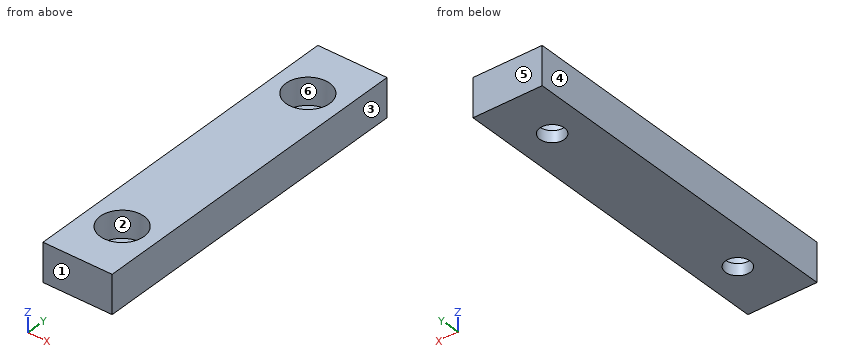
```python
from build123d import *

# Parameters (mm, degrees)
SKETCH1_W           = 44.4
SKETCH1_H           = 9
SKETCH1_R           = 2.85
BOSS_EXTRUDE1_DEPTH = 5
SKETCH1_3_R         = 2.85
SKETCH1_3_R_2       = 1.6
BOSS_EXTRUDE2_DEPTH = 1.5


with BuildPart() as part:
    # Sketch1 → Boss-Extrude1 (new body)
    with BuildSketch(Plane(origin=(0, 0, 0), x_dir=(0, 1, 0), z_dir=(0, 0, 1))):
        Rectangle(SKETCH1_W, SKETCH1_H)
        with Locations((15, 0)):
            Circle(SKETCH1_R, mode=Mode.SUBTRACT)
        with Locations((-15, 0)):
            Circle(SKETCH1_R, mode=Mode.SUBTRACT)
    extrude(amount=BOSS_EXTRUDE1_DEPTH)

    # Sketch1_3 → Boss-Extrude2 (add)
    with BuildSketch(Plane(origin=(0, 0, 0), x_dir=(0, 1, 0), z_dir=(0, 0, 1))):
        with Locations((15, 0)):
            Circle(SKETCH1_3_R)
        with Locations((15, 0)):
            Circle(SKETCH1_3_R_2, mode=Mode.SUBTRACT)
        with Locations((-15, 0)):
            Circle(SKETCH1_3_R)
        with Locations((-15, 0)):
            Circle(SKETCH1_3_R_2, mode=Mode.SUBTRACT)
    extrude(amount=BOSS_EXTRUDE2_DEPTH)


solid = part.part
```
Check sheet for the modelled part. Datum: model origin and axes. Units: mm. Face numbers are marked on the shaded views. A direction names the side the tool comes from. Give positions to 0.01 mm unless a question says otherwise; leave off trailing zeros. Write each loop counter-clockwise with the first axis right and the second up, starting at its lowest first coordinate (ties: lowest second). Pieces come first, ordered by that corner, then holes. Notation, with made-up numbers: (8, 55) - (54, 55) arc R27 ccw to (54, 88) - close; hole circle Ø3 at (31, 10.25). An arc over 180 degrees is marked (long way). Answer as a JSON object with one key per item and string values. Group by question number.
1) Depth check by flat-ended pin: P1, Ø3, axis at x = -1, y = -15, coming from the +Z side. Enter the tip coordinate at first touch or a pass-through.
2) Sectioned sample at C-C (z = 2.6). Record the cut outline in (x, y).
3) Thickness scan on probe 1 along Y at (x, z) = (0, 4.1); probe 2 along Y at (x, z) = (0, 0.8); probe 3 along X at (y, z) = (-15, 1.15). Record the ranges inside material, lowest first. Write a range as from..to.
4) Sectioned sample at B-B (y = 15). Record the cut outline in (x, z), then the cut area to 4 significant figures.
5) Access from +Z, -Z, +X, -X, +Y, -Y to the whole of each face (thin tool, end or side, straight path). Record for the marked faces 5 and 6.
6) Release check for a two-part mould opening along X. For the marked faces 1, 2, 3 and 4 record: pulls with the +X half, pulls with the -X half, needs draft (parallel to the pull), parting line crosses it, or undercut.
7) Sectioned sample at D-D (y = -14.5). Record the cut outline in (x, z), then the cut area to 3 significant figures.
8) Sectioned sample at A-A (x = 0). Record the cut outline in (y, z), then the cut area to 4 significant figures.
Geometry results:
{
 "1": {"P1": "stops at z = 1.5"},
 "2": {"outline": "(-4.5, -22.2) - (4.5, -22.2) - (4.5, 22.2) - (-4.5, 22.2) - close; hole circle Ø5.7 at (0, -15); hole circle Ø5.7 at (0, 15)"},
 "3": {"probe 1": "y = -22.2..-17.85, -12.15..12.15, 17.85..22.2", "probe 2": "y = -22.2..-16.6, -13.4..13.4, 16.6..22.2", "probe 3": "x = -4.5..-1.6, 1.6..4.5"},
 "4": {"outline": "(-4.5, 0) - (-1.6, 0) - (-1.6, 1.5) - (-2.85, 1.5) - (-2.85, 5) - (-4.5, 5) - close; (1.6, 0) - (4.5, 0) - (4.5, 5) - (2.85, 5) - (2.85, 1.5) - (1.6, 1.5) - close", "area": "20.25 mm^2"},
 "5": {"face 5": "+Z, -Z, +X, -X, +Y", "face 6": "+Z"},
 "6": {"face 1": "needs draft", "face 2": "undercut", "face 3": "pulls with the +X half", "face 4": "pulls with the -X half"},
 "7": {"outline": "(-4.5, 0) - (-1.52, 0) - (-1.52, 1.5) - (-2.81, 1.5) - (-2.81, 5) - (-4.5, 5) - close; (1.52, 0) - (4.5, 0) - (4.5, 5) - (2.81, 5) - (2.81, 1.5) - (1.52, 1.5) - close", "area": "20.8 mm^2"},
 "8": {"outline": "(-22.2, 0) - (-16.6, 0) - (-16.6, 1.5) - (-17.85, 1.5) - (-17.85, 5) - (-22.2, 5) - close; (-13.4, 0) - (13.4, 0) - (13.4, 1.5) - (12.15, 1.5) - (12.15, 5) - (-12.15, 5) - (-12.15, 1.5) - (-13.4, 1.5) - close; (16.6, 0) - (22.2, 0) - (22.2, 5) - (17.85, 5) - (17.85, 1.5) - (16.6, 1.5) - close", "area": "172.5 mm^2"}
}
